Verification items for the finished model (mm, model axes). A direction names the side the tool comes from. Give positions to 0.01 mm unless a question says otherwise; leave off trailing zeros. Loops run counter-clockwise (first coordinate to the right, second up) from the corner with the lowest first, then second, coordinate; pieces in that order, holes last. Notation, with made-up numbers: M 35,18 L 58,18 A6 cw 58,26 Z; hole C 40,41 d11. An arc over 180 degrees is marked long. Answer in a Markdown table with one row per item.
```python
from build123d import *

# Parameters (mm, degrees)
SKETCH1_W                   = 12.6
SKETCH1_H                   = 25
BOSS_EXTRUDE1_DEPTH         = 10
CUT_EXTRUDE1_START          = -4.8
SKETCH2_W                   = 7
SKETCH2_H                   = 5.8
CUT_EXTRUDE1_DEPTH          = 23.853028767
SKETCH3_W                   = 20.2
SKETCH3_H                   = 5.8
CUT_EXTRUDE2_DEPTH          = 18.47140521
SKETCH6_R                   = 1
CUT_EXTRUDE5_DEPTH          = 17.122654868
TAP_DRILL_FOR_M2X0_4_TAP1_D = 1.6
CUT_EXTRUDE6_DEPTH          = 17.122654868
CUT_EXTRUDE6_DEPTH_BACK     = 17.122654868
SKETCH9_W                   = 7
SKETCH9_H                   = 12
FILLET1_R                   = 2
SKETCH4_R                   = 1.875
CUT_EXTRUDE7_DEPTH          = 24.403632197
TAP_DRILL_FOR_M2X0_4_TAP4_D = 1.6
FILLET3_R                   = 0.2


with BuildPart() as part:
    # Sketch1 → Boss-Extrude1 (new body)
    with BuildSketch(Plane(origin=(0, 0, 0), x_dir=(1, 0, 0), z_dir=(0, 1, 0))):
        Rectangle(SKETCH1_W, SKETCH1_H)
    extrude(amount=BOSS_EXTRUDE1_DEPTH)

    # Sketch2 → Cut-Extrude1 (cut, through all)
    with BuildSketch(Plane.XY.offset(12.5).offset(CUT_EXTRUDE1_START)):
        with Locations((-2.8, 4.9)):
            Rectangle(SKETCH2_W, SKETCH2_H)
    extrude(amount=-CUT_EXTRUDE1_DEPTH, mode=Mode.SUBTRACT)

    # Sketch3 → Cut-Extrude2 (cut, through all)
    with BuildSketch(Plane.ZY.offset(-0.7)):
        with Locations((-2.4, 4.9)):
            Rectangle(SKETCH3_W, SKETCH3_H)
    extrude(amount=-CUT_EXTRUDE2_DEPTH, mode=Mode.SUBTRACT)

    # Sketch6 → Cut-Extrude5 (cut, through all)
    with BuildSketch(Plane(origin=(0, 2, 0), x_dir=(1, 0, 0), z_dir=(0, 1, 0))):
        with Locations(Location((3.15, 11, 0), (0, 0, 270))):
            Circle(SKETCH6_R)
        with Locations(Location((-3.35, 11, 0), (0, 0, 270))):
            Circle(SKETCH6_R)
    extrude(amount=-CUT_EXTRUDE5_DEPTH, mode=Mode.SUBTRACT)

    # Tap Drill for M2x0.4 Tap1 (through all)
    with Locations(Plane(origin=(3.15, 10, -11), x_dir=(0, 0, 1), z_dir=(0, 1, 0))):
        with Locations((0, 0), (0, -6.5)):
            Hole(TAP_DRILL_FOR_M2X0_4_TAP1_D / 2)

    # Sketch9 → Cut-Extrude6 (cut, two sides: drawn at the far end of the back side and taken through both)
    with BuildSketch(Plane(origin=(0, 2, 0), x_dir=(1, 0, 0), z_dir=(0, 1, 0)).offset(-CUT_EXTRUDE6_DEPTH_BACK)):
        with Locations((-2.8, -1.7)):
            Rectangle(SKETCH9_W, SKETCH9_H)
    extrude(amount=CUT_EXTRUDE6_DEPTH + CUT_EXTRUDE6_DEPTH_BACK, mode=Mode.SUBTRACT)

    # Fillet1
    fillet1_edges = [part.edges().sort_by_distance(p)[0] for p in [
        (0.7, 8.9, 7.7),
        (0.7, 1, 7.7),
        (0.7, 8.9, -4.3),
        (0.7, 1, -4.3),
    ]]
    fillet(fillet1_edges, radius=FILLET1_R)

    # Sketch4 → Cut-Extrude7 (cut, through all)
    with BuildSketch(Plane(origin=(0, 0, 7.7), x_dir=(-1, 0, 0), z_dir=(0, 0, -1))):
        with Locations((-3.5, 4.9)):
            Circle(SKETCH4_R)
    extrude(amount=-CUT_EXTRUDE7_DEPTH, mode=Mode.SUBTRACT)

    # Tap Drill for M2x0.4 Tap4 (through all)
    with Locations(Plane(origin=(-2.8, 10, 10), x_dir=(0, 0, 1), z_dir=(0, 1, 0))):
        with Locations((0, 0)):
            Hole(TAP_DRILL_FOR_M2X0_4_TAP4_D / 2)

    # Fillet3
    fillet3_edges = [part.edges().sort_by_distance(p)[0] for p in [
        (2.5, 7.8, 7.7),
        (2.5, 2, 7.7),
    ]]
    fillet(fillet3_edges, radius=FILLET3_R)


solid = part.part
```
Item 1: Tool access check on faces 1 (the flat face through (-1, 5, 7.7)), 2 (the flat face through (1, 7.8, -5)), 3 (the flat face through (-4, 9, -4.3)). Record the directions out of +Z, -Z, +X, -X, +Y, -Y that give a thin tool (end or side, any length) a straight path to the whole face; none if there is none.
Reported:
| item | result |
|---|---|
| face 1 | -X |
| face 2 | -Z, +X, -X |
| face 3 | -X, +Y, -Y |
Item 2: Sectioned sample at C-C (z = -5). Record the cut outline in (x, y), and give its area (3 significant figures).
Reported:
| item | result |
|---|---|
| outline | M -6.3,0 L 6.3,0 L 6.3,2 L -6.3,2 Z; M -6.3,7.8 L 6.3,7.8 L 6.3,10 L -6.3,10 Z |
| area | 52.9 mm^2 |
Item 3: Release check for a two-part mould opening along X. For faces 4 (the flat face through (0, 1, -12.5)), 5 (the cylindrical face through (3.91, 3.07, 10.07)), 6 (the cylindrical face through (0.1, 8.92, -3.73)) record: released by +X, released by -X, zero draft, split by the parting line, or undercut.
Reported:
| item | result |
|---|---|
| face 4 | zero draft |
| face 5 | undercut |
| face 6 | released by -X |
Item 4: Sectioned sample at D-D (x = -5). Record the cut outline in (y, z), and give its area (3 significant figures).
Reported:
| item | result |
|---|---|
| outline | M 0,-12.5 L 2,-12.5 L 2,-4.3 L 0,-4.3 Z; M 0,7.7 L 10,7.7 L 10,12.5 L 0,12.5 Z; M 7.8,-12.5 L 10,-12.5 L 10,-4.3 L 7.8,-4.3 Z |
| area | 82.4 mm^2 |
Item 5: Sectioned sample at A-A (z = 10). Record the cut outline in (x, y) (3 decimals), and give its area (3 significant figures).
Reported:
| item | result |
|---|---|
| outline | M -6.3,0 L -3.6,0 L -3.6,10 L -6.3,10 Z; M -2,0 L 6.3,0 L 6.3,10 L -2,10 Z; hole C 3.5,4.9 d3.75 |
| area | 99.0 mm^2 |
Item 6: Scan lines: L1, parallel to X at y = 0.7, z = -11; L2, parallel to X at y = 8.9, z = -11; L3, parallel to Y at x = 3.5, z = 10.75 (3 decimals). Record each from-to range of solid material in increasing order. Write a range as [from, to].
Reported:
| item | result |
|---|---|
| L1 | x = [-6.3, -4.35], [-2.35, 2.15], [4.15, 6.3] |
| L2 | x = [-6.3, -4.15], [-2.55, 2.35], [3.95, 6.3] |
| L3 | y = [0, 3.025], [6.775, 10] |
Item 7: Go/stop test with flat-tipped pins: pin 1 (1.8 mm diameter, centred on x = 3.15, z = -11, fed in from -Y); pin 2 (5 mm diameter, centred on x = 3.5, y = 4.9, fed in from -Z); pin 3 (1.8 mm diameter, centred on y = 8.5, z = 0, fed in from -X). Record where each tip stops, or that it passes through.
Reported:
| item | result |
|---|---|
| pin 1 | stops at y = 7.8 |
| pin 2 | stops at z = 7.7 |
| pin 3 | stops at x = 0.7 |
Item 8: Sectioned sample at B-B (y = 8.25). Record the cut outline in (x, z).
Reported:
| item | result |
|---|---|
| outline | M -6.3,-12.5 L 6.3,-12.5 L 6.3,12.5 L -6.3,12.5 L -6.3,7.7 L -1.3,7.7 A2 cw 0.7,5.7 L 0.7,-2.3 A2 cw -1.3,-4.3 L -6.3,-4.3 Z; hole C -3.35,-11 d1.6; hole C -2.8,10 d1.6; hole C 3.15,-11 d1.6 |
